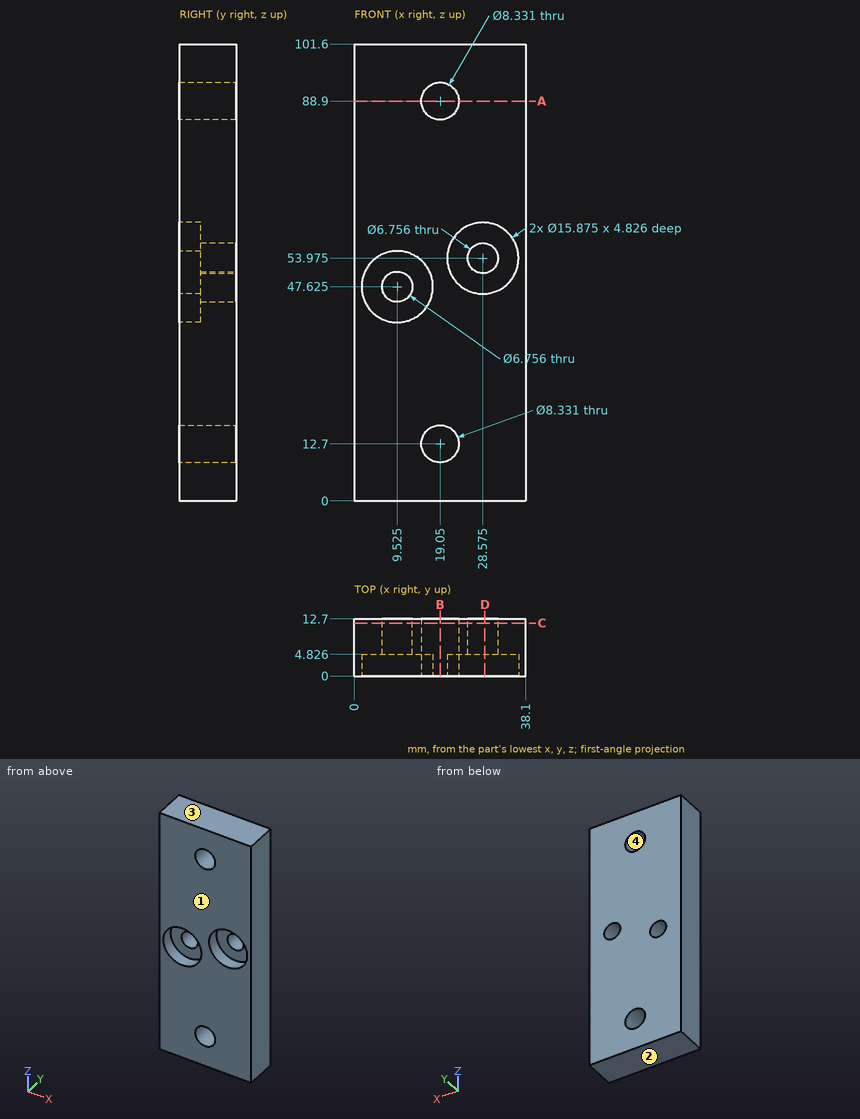
Here's the drawing with two shaded views (mm, measured from the low corner). I have some questions. Give positions to 0.01 mm unless a question says otherwise; leave off trailing zeros. Loops run counter-clockwise (first coordinate to the right, second up) from the corner with the lowest first, then second, coordinate; pieces in that order, holes last. Notation, with made-up numbers: M 87.5,54.25 L 126.5,54.25 A25 ccw 126.5,78.25 Z; hole C 68.25,9.5 d10. An arc over 180 degrees is marked long. Use one line per item in the form item = value. Start each with the question number.
(1) I want a section at D-D, the plane x = 29. Write out the boundary of the cut face in (y, z), and give its area (3 significant figures).
(2) Thinking about a two-plate mould opening in Z: for the marked faces 1, 2, 3 and 4, which applies, released by +Z, released by -Z, zero draft, split by the parting line, or undercut?
(3) I want a section at A-A, the plane z = 88.9. Write out the boundary of the cut face in (x, y) (1 decimal), and give its area (3 significant figures).
(4) I'm going to push flat-ended pins straight in: P1, Ø9.5, axis at x = 9.525, z = 47.625, coming from the -Y side; P2, Ø5.5, axis at x = 28.575, z = 53.975, coming from the +Y side. Where does each tip first touch, or does it pass through?
(5) I want a section at C-C, the plane y = 11.75. State how many separate pieces and enclosed holes the cut face has, and give its area (3 significant figures).
(6) I want a section at B-B, the plane x = 19.05. Write out the boundary of the cut face in (y, z) (1 decimal), and give its area (3 significant figures).
(7) Please list where these lines run through material, in increasing order: line 1 (X direction, y = 9, z = 12.7) (1 decimal); line 2 (X direction, y = 7.75, z = 54); line 3 (Z direction, x = 22, y = 10.5).
Worked out:
q1.outline = M 0,0 L 12.7,0 L 12.7,50.62 L 4.83,50.62 L 4.83,46.05 L 0,46.05 Z; M 0,61.9 L 4.83,61.9 L 4.83,57.33 L 12.7,57.33 L 12.7,101.6 L 0,101.6 Z
q1.area = 1,160 mm²
q2.face_1 = zero draft
q2.face_2 = released by -Z
q2.face_3 = released by +Z
q2.face_4 = undercut
q3.outline = M 0,0 L 14.9,0 L 14.9,12.7 L 0,12.7 Z; M 23.2,0 L 38.1,0 L 38.1,12.7 L 23.2,12.7 Z
q3.area = 378 mm²
q4.P1 = 4.83
q4.P2 = through
q5.separate_pieces = 1
q5.enclosed_holes = 4
q5.area = 3,690 mm²
q6.outline = M 0,0 L 12.7,0 L 12.7,8.5 L 0,8.5 Z; M 0,16.9 L 12.7,16.9 L 12.7,84.7 L 0,84.7 Z; M 0,93.1 L 12.7,93.1 L 12.7,101.6 L 0,101.6 Z
q6.area = 1,080 mm²
q7.line_1 = 0 to 14.9, 23.2 to 38.1
q7.line_2 = 0 to 25.2, 31.95 to 38.1
q7.line_3 = 0 to 9.76, 15.64 to 85.96, 91.84 to 101.6
